Input: part model. Units: mm. Frame: model coordinates. A direction names the side the tool comes from. Round coordinates to 2 decimals unless told otherwise and drop trailing zeros. Write each loop counter-clockwise with the first axis right and the second up, starting at its lowest first coordinate (ties: lowest second). Pieces come first, ordered by that corner, then holes. Notation, with made-up numbers: (0, 40.5) -> (34, 40.5) arc R20 ccw to (34, 53.5) -> close; hole circle Ø1 at (-38, 39). An arc over 180 degrees is marked (long way). Write item = value, one per line.
```python
from build123d import *

# Parameters (mm, degrees)
SKETCH1_R             = 3
BOSS_EXTRUDE1_DEPTH   = 2.65
SKETCH1_R_2           = 4.425
SKETCH1_R_3           = 1
BOSS_EXTRUDE1_2_DEPTH = 2.65
SKETCH1_4_R           = 4.425
SKETCH1_4_R_2         = 3
BOSS_EXTRUDE2_DEPTH   = 6
SKETCH2_R             = 4.5
SKETCH2_R_2           = 3.5
SKETCH2_R_3           = 3.25
SKETCH2_R_4           = 3
SKETCH2_R_5           = 1.75
CUT_EXTRUDE1_DEPTH    = 0.2
SKETCH2_4_R           = 3.5
SKETCH2_4_R_2         = 3.25
BOSS_EXTRUDE3_DEPTH   = 0.5
CUT_EXTRUDE2_REACH    = 79.29
SKETCH2_5_R           = 1.75


with BuildPart() as part:
    # Sketch1 → Boss-Extrude1 (new body)
    with BuildSketch(Plane(origin=(0, 0, 0), x_dir=(1, 0, 0), z_dir=(0, 1, 0))):
        with Locations(Location((-36.075458566, -36.896070591, 0), (0, 0, 270))):
            Circle(SKETCH1_R)
    extrude(amount=BOSS_EXTRUDE1_DEPTH)


with BuildPart() as body_2:
    # Sketch1 → Boss-Extrude1 2 (new body)
    with BuildSketch(Plane(origin=(0, 0, 0), x_dir=(1, 0, 0), z_dir=(0, 1, 0))):
        with BuildLine():
            Line((-30.457637809, -32.471070591), (-30.650458566, -32.471070591))
            ThreePointArc((-30.650458566, -32.471070591), (-31.357565348, -32.178177373), (-31.650458566, -31.471070591))
            Line((-31.650458566, -31.471070591), (-31.650458566, -31.278249834))
            ThreePointArc((-31.650458566, -31.278249834), (-31.744632332, -29.909087094), (-32.025379888, -28.565712196))
            Line((-32.025379888, -28.565712196), (-34.391069798, -20.171376505))
            ThreePointArc((-34.391069798, -20.171376505), (-36.075458566, -18.896070591), (-37.759847335, -20.171376505))
            Line((-37.759847335, -20.171376505), (-40.125537245, -28.565712196))
            ThreePointArc((-40.125537245, -28.565712196), (-40.406284801, -29.909087094), (-40.500458566, -31.278249834))
            Line((-40.500458566, -31.278249834), (-40.500458566, -31.471070591))
            ThreePointArc((-40.500458566, -31.471070591), (-40.793351785, -32.178177373), (-41.500458566, -32.471070591))
            Line((-41.500458566, -32.471070591), (-41.693279324, -32.471070591))
            ThreePointArc((-41.693279324, -32.471070591), (-43.062442064, -32.565244357), (-44.405816962, -32.845991913))
            Line((-44.405816962, -32.845991913), (-52.800152653, -35.211681823))
            ThreePointArc((-52.800152653, -35.211681823), (-54.075458566, -36.896070591), (-52.800152653, -38.58045936))
            Line((-52.800152653, -38.58045936), (-44.405816962, -40.94614927))
            ThreePointArc((-44.405816962, -40.94614927), (-43.062442064, -41.226896826), (-41.693279324, -41.321070591))
            Line((-41.693279324, -41.321070591), (-41.500458566, -41.321070591))
            ThreePointArc((-41.500458566, -41.321070591), (-40.793351785, -41.61396381), (-40.500458566, -42.321070591))
            Line((-40.500458566, -42.321070591), (-40.500458566, -42.513891349))
            ThreePointArc((-40.500458566, -42.513891349), (-40.406284801, -43.883054089), (-40.125537245, -45.226428987))
            Line((-40.125537245, -45.226428987), (-37.759847335, -53.620764678))
            ThreePointArc((-37.759847335, -53.620764678), (-36.075458566, -54.896070591), (-34.391069798, -53.620764678))
            Line((-34.391069798, -53.620764678), (-32.025379888, -45.226428987))
            ThreePointArc((-32.025379888, -45.226428987), (-31.744632332, -43.883054089), (-31.650458566, -42.513891349))
            Line((-31.650458566, -42.513891349), (-31.650458566, -42.321070591))
            ThreePointArc((-31.650458566, -42.321070591), (-31.357565348, -41.61396381), (-30.650458566, -41.321070591))
            Line((-30.650458566, -41.321070591), (-30.457637809, -41.321070591))
            ThreePointArc((-30.457637809, -41.321070591), (-29.088475069, -41.226896826), (-27.745100171, -40.94614927))
            Line((-27.745100171, -40.94614927), (-19.35076448, -38.58045936))
            ThreePointArc((-19.35076448, -38.58045936), (-18.075458566, -36.896070591), (-19.35076448, -35.211681823))
            Line((-19.35076448, -35.211681823), (-27.745100171, -32.845991913))
            ThreePointArc((-27.745100171, -32.845991913), (-29.088475069, -32.565244357), (-30.457637809, -32.471070591))
        make_face()
        with Locations(Location((-36.075458566, -36.896070591, 0), (0, 0, 270))):
            Circle(SKETCH1_R_2, mode=Mode.SUBTRACT)
        with Locations(Location((-52.325458566, -36.896070591, 0), (0, 0, 270))):
            Circle(SKETCH1_R_3, mode=Mode.SUBTRACT)
        with Locations(Location((-49.575458566, -36.896070591, 0), (0, 0, 270))):
            Circle(SKETCH1_R_3, mode=Mode.SUBTRACT)
        with Locations(Location((-46.825458566, -36.896070591, 0), (0, 0, 270))):
            Circle(SKETCH1_R_3, mode=Mode.SUBTRACT)
        with Locations(Location((-44.075458566, -36.896070591, 0), (0, 0, 270))):
            Circle(SKETCH1_R_3, mode=Mode.SUBTRACT)
        with Locations(Location((-28.075458566, -36.896070591, 0), (0, 0, 270))):
            Circle(SKETCH1_R_3, mode=Mode.SUBTRACT)
        with Locations(Location((-25.325458566, -36.896070591, 0), (0, 0, 270))):
            Circle(SKETCH1_R_3, mode=Mode.SUBTRACT)
        with Locations(Location((-22.575458566, -36.896070591, 0), (0, 0, 270))):
            Circle(SKETCH1_R_3, mode=Mode.SUBTRACT)
        with Locations(Location((-19.825458566, -36.896070591, 0), (0, 0, 270))):
            Circle(SKETCH1_R_3, mode=Mode.SUBTRACT)
        with Locations(Location((-36.075458566, -20.646070591, 0), (0, 0, 270))):
            Circle(SKETCH1_R_3, mode=Mode.SUBTRACT)
        with Locations(Location((-36.075458566, -23.396070591, 0), (0, 0, 270))):
            Circle(SKETCH1_R_3, mode=Mode.SUBTRACT)
        with Locations(Location((-36.075458566, -26.146070591, 0), (0, 0, 270))):
            Circle(SKETCH1_R_3, mode=Mode.SUBTRACT)
        with Locations(Location((-36.075458566, -28.896070591, 0), (0, 0, 270))):
            Circle(SKETCH1_R_3, mode=Mode.SUBTRACT)
        with Locations(Location((-36.075458566, -44.896070591, 0), (0, 0, 270))):
            Circle(SKETCH1_R_3, mode=Mode.SUBTRACT)
        with Locations(Location((-36.075458566, -47.646070591, 0), (0, 0, 270))):
            Circle(SKETCH1_R_3, mode=Mode.SUBTRACT)
        with Locations(Location((-36.075458566, -50.396070591, 0), (0, 0, 270))):
            Circle(SKETCH1_R_3, mode=Mode.SUBTRACT)
        with Locations(Location((-36.075458566, -53.146070591, 0), (0, 0, 270))):
            Circle(SKETCH1_R_3, mode=Mode.SUBTRACT)
    extrude(amount=BOSS_EXTRUDE1_2_DEPTH)

    # Sketch1_4 → Boss-Extrude2 (add)
    with BuildSketch(Plane(origin=(0, 0, 0), x_dir=(1, 0, 0), z_dir=(0, 1, 0))):
        with Locations(Location((-36.075458566, -36.896070591, 0), (0, 0, 270))):
            Circle(SKETCH1_4_R)
        with Locations(Location((-36.075458566, -36.896070591, 0), (0, 0, 270))):
            Circle(SKETCH1_4_R_2, mode=Mode.SUBTRACT)
    extrude(amount=BOSS_EXTRUDE2_DEPTH)


with BuildPart() as cut_extrude1_tool:
    # Sketch2 → Cut-Extrude1 (new body)
    with BuildSketch(Plane.XZ):
        with Locations(Location((-36.075458566, 36.896070591, 0), (0, 0, 270))):
            Circle(SKETCH2_R)
        with Locations(Location((-36.075458566, 36.896070591, 0), (0, 0, 270))):
            Circle(SKETCH2_R_2, mode=Mode.SUBTRACT)
        with Locations(Location((-36.075458566, 36.896070591, 0), (0, 0, 270))):
            Circle(SKETCH2_R_3)
        with Locations(Location((-36.075458566, 36.896070591, 0), (0, 0, 270))):
            Circle(SKETCH2_R_4, mode=Mode.SUBTRACT)
        with Locations(Location((-36.075458566, 36.896070591, 0), (0, 0, 270))):
            Circle(SKETCH2_R_4)
        with Locations(Location((-36.075458566, 36.896070591, 0), (0, 0, 270))):
            Circle(SKETCH2_R_5, mode=Mode.SUBTRACT)
    extrude(amount=-CUT_EXTRUDE1_DEPTH)


with BuildPart() as part_1:
    add(part.part)

    # Cut-Extrude1: cut by cut_extrude1_tool
    add(cut_extrude1_tool.part, mode=Mode.SUBTRACT)


with BuildPart() as body_2_1:
    add(body_2.part)

    # Cut-Extrude1: cut by cut_extrude1_tool
    add(cut_extrude1_tool.part, mode=Mode.SUBTRACT)


    add(part_1.part)  # Boss-Extrude3 merges part
    # Sketch2_4 → Boss-Extrude3 (add)
    with BuildSketch(Plane.XZ):
        with Locations(Location((-36.075458566, 36.896070591, 0), (0, 0, 270))):
            Circle(SKETCH2_4_R)
        with Locations(Location((-36.075458566, 36.896070591, 0), (0, 0, 270))):
            Circle(SKETCH2_4_R_2, mode=Mode.SUBTRACT)
    extrude(amount=BOSS_EXTRUDE3_DEPTH)

    # Sketch2_5 → Cut-Extrude2 (cut, up to next)
    with BuildSketch(Plane.XZ, mode=Mode.PRIVATE) as cut_extrude2_sk1:
        with Locations(Location((-36.075458566, 36.896070591, 0), (0, 0, 270))):
            Circle(SKETCH2_5_R)
    cut_extrude2_tool1 = extrude(cut_extrude2_sk1.sketch, amount=-CUT_EXTRUDE2_REACH, mode=Mode.PRIVATE) & body_2_1.part
    add(cut_extrude2_tool1.solids().sort_by_distance((-36.075459, 0, 36.896071))[0], mode=Mode.SUBTRACT)


solid = body_2_1.part
```
1) First-contact query: P1, Ø2.5, axis at x = -36.08, z = 28.9, coming from the -Y side; P2, Ø1, axis at y = 5, z = 39.5, coming from the +X side; P3, Ø2.5, axis at x = -36.08, z = 50.4, coming from the +Y side. Flat tips, straight axial feed; report the tip coordinate or a pass-through.
Solutions:
P1 = 0
P2 = -32.18
P3 = 2.65
2) Cut plane A-A (z = 26). Return the cut outline in (x, y).
Solutions:
outline = (-39.4, 0) -> (-37.06, 0) -> (-37.06, 2.65) -> (-39.4, 2.65) -> close; (-35.09, 0) -> (-32.75, 0) -> (-32.75, 2.65) -> (-35.09, 2.65) -> close
3) Line query: L1, parallel to Y at x = -33, z = 45; L2, parallel to Z at x = -30.5, y = 1.5; L3, parallel to Z at x = -24, y = 2.5. Output: solid intervals per line, ascending. Write a range as from..to.
Solutions:
L1 = 0..2.65
L2 = 32.47..41.32
L3 = 33.9..39.89
4) Access query for faces 1 (the face through (-48.5, 1.3, 34)), 2 (the face through (-35.881, 4.302, 32.475)). Directions: +Z, -Z, +X, -X, +Y, -Y. A direction counts if a zero-diameter tool reaches every point of the face in a straight line with its end or side. Return the directions, or none.
Solutions:
face_1 = -Z, -X, +Y, -Y
face_2 = +Y
5) Cut plane D-D (x = -29.5). Return the cut outline in (y, z), and give its area (3 significant figures).
Solutions:
outline = (0, 32.52) -> (2.65, 32.52) -> (2.65, 41.28) -> (0, 41.28) -> close
area = 23.2 mm^2
6) Cut plane B-B (y = 1.5). Count the separate pieces of the cut face and the enclosed holes in it, and give its area (3 significant figures).
Solutions:
separate_pieces = 1
enclosed_holes = 17
area = 360 mm^2
7) Draft query along Z for faces 3 (the face through (-47.8, 1.31, 36.68)), 4 (the face through (-36.107, 1.306, 54.896)), 5 (the face through (-37, 0.2, 35)), 6 (the face through (-37, 6, 40)). Return one class per face: +Z half, -Z half, draft (parallel to the pull), parting line (faces both ways), or undercut.
Solutions:
face_3 = undercut
face_4 = +Z half
face_5 = undercut
face_6 = draft
8) Cut plane C-C (y = 4.75). Return the cut outline in (x, z) (3 decimals).
Solutions:
outline = circle Ø8.85 at (-36.075, 36.896); hole circle Ø6 at (-36.075, 36.896)
